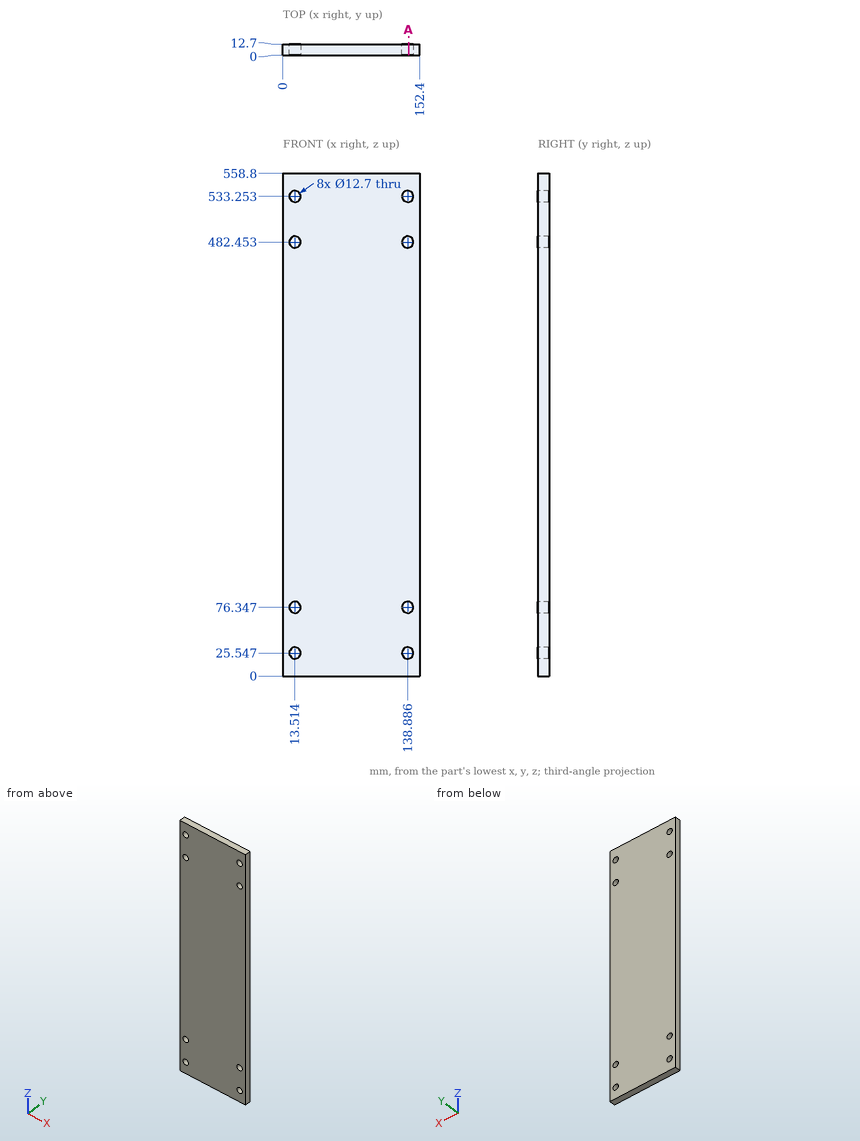
Geometry check sheet. Reference: drawing and pictorial views, mm from the part's lowest x, y, z. Coordinates: 2 decimals unless noted, no trailing zeros. Order: outer loops, then holes, each group sorted by start corner. A loop starts at its lowest first (then second) coordinate and runs counter-clockwise, first axis right, second up. Notation, with made-up numbers: (14.5, 45.5) -> (47.5, 45.5) arc R18 cw to (47.5, 65.5) -> close; hole circle Ø9 at (-9, -32). An arc over 180 degrees is marked (long way). Use CSV: the item, a comma, the result in double quotes. Start each with the question number.
Q1. Section check A-A, the plane x = 140. Record the cut outline in (y, z), and give its area (3 significant figures).
Q2. Thickness scan on line 1 along Z through (x, y) = (139.5, 6.5); line 2 along Z through (x, y) = (143.5, 5.75) (1 decimal); line 3 along X through (y, z) = (3, 477). Record the ranges inside material, lowest first.
Q3. Depth check by flat-ended pin: P1, Ø7.5, axis at x = 138.89, z = 482.45, coming from the -Y side. Enter the tip coordinate at first touch or a pass-through.
Returned:
1,outline,"(0, 0) -> (12.7, 0) -> (12.7, 19.3) -> (0, 19.3) -> close; (0, 31.8) -> (12.7, 31.8) -> (12.7, 70.1) -> (0, 70.1) -> close; (0, 82.6) -> (12.7, 82.6) -> (12.7, 476.2) -> (0, 476.2) -> close; (0, 488.7) -> (12.7, 488.7) -> (12.7, 527) -> (0, 527) -> close; (0, 539.5) -> (12.7, 539.5) -> (12.7, 558.8) -> (0, 558.8) -> close"
1,area,"6,460 mm^2"
2,line 1,"z = 0 to 19.23, 31.87 to 70.03, 82.67 to 476.13, 488.77 to 526.93, 539.57 to 558.8"
2,line 2,"z = 0 to 21.2, 29.9 to 72, 80.7 to 478.1, 486.8 to 528.9, 537.6 to 558.8"
2,line 3,"x = 0 to 10.26, 16.77 to 135.63, 142.14 to 152.4"
3,P1,"passes through"
